Geometry check sheet. Reference: the model listing, model coordinates, mm. Face numbers are marked on the shaded views. A direction names the side the tool comes from. Round coordinates to 2 decimals unless told otherwise and drop trailing zeros. Order: outer loops, then holes, each group sorted by start corner. A loop starts at its lowest first (then second) coordinate and runs counter-clockwise, first axis right, second up. Notation, with made-up numbers: (-3, 29.25) - (35, 29.25) arc R19 cw to (35, 46.25) - close; hole circle Ø10 at (-40, 72.5). An arc over 180 degrees is marked (long way). One line per question, with ' | ' between items. Start each with the question number.
Q1. Mould release check, pull along Z, two halves, no side actions. Record for the marked faces 1, 2 and 3: +Z half, -Z half, draft (parallel to the pull), parting line (faces both ways), or undercut.
Q2. Material ranges on line 1 along X through (y, z) = (-21, 16); line 2 along Z through (x, y) = (-24.5, -28); line 3 along Y through (x, z) = (3, -5), recorded low to high.
Q3. Sectioned sample at A-A, the plane z = -5. Enter the section's corners in (x, y) (3 decimals).
Q4. Gauge pin test, flat ends, axial feed: P1, Ø4.5, axis at x = 2, y = -16.5, coming from the +Z side; P2, Ø6, axis at x = 1.5, y = -11.5, coming from the -Z side; P3, Ø4, axis at x = -29.5, y = -16, coming from the +Z side. Record the tip position at first contact, or that the pin passes through.
Q5. Tool access check on the marked faces 4 and 5. Record the directions out of +Z, -Z, +X, -X, +Y, -Y that give a thin tool (end or side, any length) a straight path to the whole face; none if there is none.
Q6. Sectioned sample at B-B, the plane y = -13. Enter the section's corners in (x, z) (3 decimals).
```python
from build123d import *

# Parameters (mm, degrees)
F1_DEPTH     = 31.75
F2_R         = 3.175
F3_W         = 19.05
F3_H         = 50.8
F4_DEPTH     = 10.6367849431
F5_T4_DEPTH  = 76.9282991577
F5_T10_DEPTH = 45.1782991577
F5_T16_DEPTH = 45.1782991577
F5_T22_DEPTH = 76.9282991577


# Not quite as in the source:
# - a fillet or chamfer that OpenCascade refuses, or shapes differently, is made with other operations: its cross-section is extruded or revolved along the edge and cut away or added


with BuildPart() as f1:
    # F0 (on Front) → F1 (new body)
    with BuildSketch(Plane.XZ):
        with BuildLine():
            Line((-5.2392150569, 71.7959681749), (-24.2892150569, 71.7959681749))
            ThreePointArc((-24.2892150569, 71.7959681749), (-35.5145352082, 67.1462883263), (-40.1642150569, 55.9209681749))
            Line((-40.1642150569, 55.9209681749), (-40.1642150569, -39.3290318251))
            ThreePointArc((-40.1642150569, -39.3290318251), (-35.5145352082, -50.5543519764), (-24.2892150569, -55.2040318251))
            Line((-24.2892150569, -55.2040318251), (-5.2392150569, -55.2040318251))
            ThreePointArc((-5.2392150569, -55.2040318251), (5.9861050945, -50.5543519764), (10.6357849431, -39.3290318251))
            Line((10.6357849431, -39.3290318251), (10.6357849431, 55.9209681749))
            ThreePointArc((10.6357849431, 55.9209681749), (5.9861050945, 67.1462883263), (-5.2392150569, 71.7959681749))
        make_face()
    extrude(amount=F1_DEPTH)

    # F2
    f2_edges = [f1.edges().sort_by_distance(p)[0] for p in [
        (-24.289215, -15.875, -55.204032),
        (-5.239215, -15.875, -55.204032),
        (-14.764215, 0, -55.204032),
        (-14.764215, -31.75, -55.204032),
        (-5.239215, -15.875, 71.795968),
        (-24.289215, -15.875, 71.795968),
        (-14.764215, 0, 71.795968),
        (-14.764215, -31.75, 71.795968),
        (10.635785, 0, 8.295968),
        (10.635785, -31.75, 8.295968),
        (5.986105, 0, 67.146288),
        (5.986105, -31.75, 67.146288),
        (-35.514535, 0, 67.146288),
        (-35.514535, -31.75, 67.146288),
        (-40.164215, 0, 8.295968),
        (-40.164215, -31.75, 8.295968),
        (-35.514535, 0, -50.554352),
        (-35.514535, -31.75, -50.554352),
        (5.986105, 0, -50.554352),
        (5.986105, -31.75, -50.554352),
    ]]
    fillet(f2_edges, radius=F2_R)

    # F3 (on Right) → F4 (cut, through all)
    with BuildSketch(Plane.YZ):
        with Locations((-16.1061841063, -2.5141499803)):
            Rectangle(F3_W, F3_H)
    extrude(amount=F4_DEPTH, mode=Mode.SUBTRACT)

    # F5: chamfer of 5.08 on 4 edges, made by hand


with BuildPart() as f5_tool2:
    # F5_s3 → F5_t4 (new body)
    with BuildSketch(Plane.XY.offset(35.9499995986)):
        Polygon((10.6357849431, -30.7111841063), (5.5557849431, -25.6311841063), (10.6357849431, -25.6311841063), align=None)
    extrude(amount=-F5_T4_DEPTH)

    split(bisect_by=Plane(origin=(-11.1791825186, 0, -11.1791825186), x_dir=(0, 1, 0), z_dir=(0.7071067812, 0, 0.7071067812)), keep=Keep.TOP)

    split(bisect_by=Plane(origin=(-8.6650325383, 0, 8.6650325383), x_dir=(0, 1, 0), z_dir=(0.7071067812, 0, -0.7071067812)), keep=Keep.TOP)


with BuildPart() as f1_1:
    add(f1.part)

    # F5_t1: cut F5_tool2
    add(f5_tool2.part, mode=Mode.SUBTRACT)


with BuildPart() as f5_tool8:
    # F5_s9 → F5_t10 (new body)
    with BuildSketch(Plane.XZ.offset(-6.4829654725)):
        Polygon((10.6357849431, 27.9658500197), (5.5557849431, 22.8858500197), (10.6357849431, 22.8858500197), align=None)
    extrude(amount=F5_T10_DEPTH)

    split(bisect_by=Plane(origin=(-10.0376995816, -10.0376995816, 0), x_dir=(0, 0, 1), z_dir=(0.7071067812, 0.7071067812, 0)), keep=Keep.TOP)

    split(bisect_by=Plane(origin=(6.0684845247, -6.0684845247, 0), x_dir=(0, 0, 1), z_dir=(0.7071067812, -0.7071067812, 0)), keep=Keep.TOP)


with BuildPart() as f1_2:
    add(f1_1.part)

    # F5_t7: cut F5_tool8
    add(f5_tool8.part, mode=Mode.SUBTRACT)


with BuildPart() as f5_tool14:
    # F5_s15 → F5_t16 (new body)
    with BuildSketch(Plane.XZ.offset(38.6953336852)):
        Polygon((10.6357849431, -32.9941499803), (5.5557849431, -27.9141499803), (10.6357849431, -27.9141499803), align=None)
    extrude(amount=-F5_T16_DEPTH)

    split(bisect_by=Plane(origin=(-10.0376995816, -10.0376995816, 0), x_dir=(0, 0, 1), z_dir=(0.7071067812, 0.7071067812, 0)), keep=Keep.TOP)

    split(bisect_by=Plane(origin=(6.0684845247, -6.0684845247, 0), x_dir=(0, 0, 1), z_dir=(0.7071067812, -0.7071067812, 0)), keep=Keep.TOP)


with BuildPart() as f1_3:
    add(f1_2.part)

    # F5_t13: cut F5_tool14
    add(f5_tool14.part, mode=Mode.SUBTRACT)


with BuildPart() as f5_tool20:
    # F5_s21 → F5_t22 (new body)
    with BuildSketch(Plane.XY.offset(-40.9782995592)):
        Polygon((10.6357849431, -1.5011841063), (5.5557849431, -6.5811841063), (10.6357849431, -6.5811841063), align=None)
    extrude(amount=F5_T22_DEPTH)

    split(bisect_by=Plane(origin=(-11.1791825186, 0, -11.1791825186), x_dir=(0, 1, 0), z_dir=(0.7071067812, 0, 0.7071067812)), keep=Keep.TOP)

    split(bisect_by=Plane(origin=(-8.6650325383, 0, 8.6650325383), x_dir=(0, 1, 0), z_dir=(0.7071067812, 0, -0.7071067812)), keep=Keep.TOP)


with BuildPart() as f1_4:
    add(f1_3.part)

    # F5_t19: cut F5_tool20
    add(f5_tool20.part, mode=Mode.SUBTRACT)


solid = f1_4.part
```
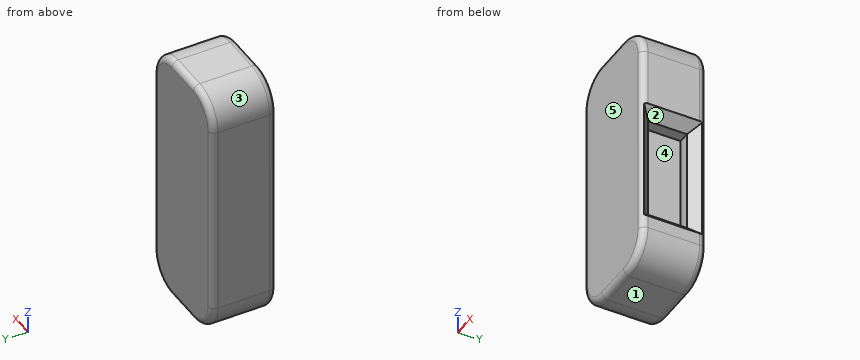
Determined:
1) face 1: -Z half | face 2: undercut | face 3: +Z half
2) line 1: x = -40.16 to 0 | line 2: z = -55.2 to 71.79 | line 3: y = -31.75 to -25.63, -6.58 to 0
3) outline: (-40.164, -28.575) arc R3.175 ccw to (-36.989, -31.75) - (7.461, -31.75) arc R3.175 ccw to (10.164, -30.24) - (5.556, -25.631) - (0, -25.631) - (0, -6.581) - (5.556, -6.581) - (10.327, -1.81) arc R3.175 ccw to (7.461, 0) - (-36.989, 0) arc R3.175 ccw to (-40.164, -3.175) - close
4) P1: stops at z = 70.99 | P2: stops at z = -54.76 | P3: stops at z = 71.47
5) face 4: +X | face 5: +Z, -Z, +X, -X, -Y
6) outline: (-40.164, -39.329) arc R15.875 ccw to (-24.289, -55.204) - (-5.239, -55.204) arc R15.875 ccw to (10.636, -39.329) - (10.636, -32.994) - (5.556, -27.914) - (0, -27.914) - (0, 22.886) - (5.556, 22.886) - (10.636, 27.966) - (10.636, 55.921) arc R15.875 ccw to (-5.239, 71.796) - (-24.289, 71.796) arc R15.875 ccw to (-40.164, 55.921) - close
